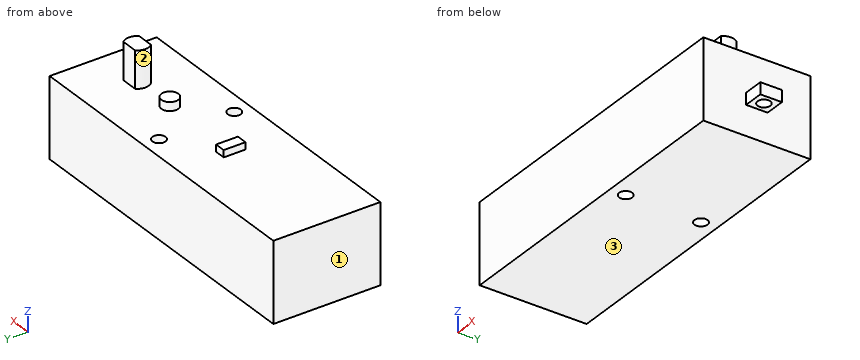
```python
from build123d import *

# Parameters (mm, degrees)
SKETCH1_W           = 75.1586
SKETCH1_H           = 25.1968
BOSS_EXTRUDE1_DEPTH = 18.7452
SKETCH2_W           = 4.8006
SKETCH2_H           = 5.08
BOSS_EXTRUDE2_DEPTH = 2.7432
SKETCH4_R           = 1.4986
CUT_EXTRUDE1_DEPTH  = 85.400741157
SKETCH3_R           = 1.9939
BOSS_EXTRUDE3_DEPTH = 2.032
SKETCH5_R           = 2.7051
BOSS_EXTRUDE4_DEPTH = 8.6614
CUT_EXTRUDE2_START  = -8.6614
CUT_EXTRUDE2_DEPTH  = 8.6614
SKETCH7_R           = 1.5367
CUT_EXTRUDE3_DEPTH  = 86.905383521
SKETCH8_W           = 2.54
SKETCH8_H           = 5.1308
BOSS_EXTRUDE5_DEPTH = 1.651


with BuildPart() as part:
    # Sketch1 → Boss-Extrude1 (new body)
    with BuildSketch(Plane.XY):
        with Locations((37.5793, 12.5984)):
            Rectangle(SKETCH1_W, SKETCH1_H)
    extrude(amount=BOSS_EXTRUDE1_DEPTH)

    # Sketch2 → Boss-Extrude2 (add)
    with BuildSketch(Plane.XY.offset(7.0104)):
        with Locations((77.5589, 12.5984)):
            Rectangle(SKETCH2_W, SKETCH2_H)
    extrude(amount=BOSS_EXTRUDE2_DEPTH)

    # Sketch4 → Cut-Extrude1 (cut, through all)
    with BuildSketch(Plane.XY.offset(9.7536)):
        with Locations((77.5589, 12.5984)):
            Circle(SKETCH4_R)
    extrude(amount=-CUT_EXTRUDE1_DEPTH, mode=Mode.SUBTRACT)

    # Sketch3 → Boss-Extrude3 (add)
    with BuildSketch(Plane.XY.offset(18.7452)):
        with Locations(Location((52.7431, 12.5984, 0), (0, 0, 180))):
            Circle(SKETCH3_R)
    extrude(amount=BOSS_EXTRUDE3_DEPTH)

    # Sketch5 → Boss-Extrude4 (add)
    with BuildSketch(Plane.XY.offset(18.7452)):
        with Locations(Location((63.7413, 12.5984, 0), (0, 0, 180))):
            Circle(SKETCH5_R)
    extrude(amount=BOSS_EXTRUDE4_DEPTH)

    # Sketch6 → Cut-Extrude2 (cut)
    with BuildSketch(Plane.XY.offset(27.4066).offset(CUT_EXTRUDE2_START)):
        with BuildLine():
            ThreePointArc((65.710946763, 14.4526), (63.7413, 15.3035), (61.771653237, 14.4526))
            Line((61.771653237, 14.4526), (65.710946763, 14.4526))
        make_face()
        with BuildLine():
            Line((65.710946763, 10.7442), (61.771653237, 10.7442))
            ThreePointArc((61.771653237, 10.7442), (63.7413, 9.8933), (65.710946763, 10.7442))
        make_face()
    extrude(amount=CUT_EXTRUDE2_DEPTH, mode=Mode.SUBTRACT)

    # Sketch7 → Cut-Extrude3 (cut, through all)
    with BuildSketch(Plane.XY.offset(18.7452)):
        with Locations((43.7515, 21.463)):
            Circle(SKETCH7_R)
        with Locations((43.7515, 3.7338)):
            Circle(SKETCH7_R)
    extrude(amount=-CUT_EXTRUDE3_DEPTH, mode=Mode.SUBTRACT)

    # Sketch8 → Boss-Extrude5 (add)
    with BuildSketch(Plane.XY.offset(18.7452)):
        with Locations((32.2707, 12.5984)):
            Rectangle(SKETCH8_W, SKETCH8_H)
    extrude(amount=BOSS_EXTRUDE5_DEPTH)


solid = part.part
```
Geometry check sheet. Reference: the model listing, model coordinates, mm. Face numbers are marked on the shaded views. Give positions to 0.01 mm unless a question says otherwise; leave off trailing zeros. Order: outer loops, then holes, each group sorted by start corner. A loop starts at its lowest first (then second) coordinate and runs counter-clockwise, first axis right, second up.
1. Section check B-B, the plane y = 20.75. Enter the section's corners in (x, z).
2. Release check for a two-part mould opening along X. For the marked faces 1, 2 and 3 record: pulls with the +X half, pulls with the -X half, needs draft (parallel to the pull), parting line crosses it, or undercut.
3. Section check A-A, the plane x = 65. Enter the section's corners in (y, z), and give its area (3 significant figures).
4. Section check D-D, the plane y = 16.5. Enter the section's corners in (x, z).
5. Gauge pin test, flat ends, axial feed: pin 1 Ø4 at (x, y) = (78, 13.5) entering from -Z; pin 2 Ø3 at (x, z) = (78.5, 9) entering from +Y; pin 3 Ø0.8 at (x, z) = (32, 20) entering from -Y; pin 4 Ø6 at (y, z) = (6.5, 10) entering from -X. Record the tip position at first contact, or that the pin passes through.
6. Thickness scan on L1, parallel to X at y = 7, z = 13; L2, parallel to Y at x = 62, z = 25.75; L3, parallel to Z at x = 28, y = 21. Record the ranges inside material, lowest first.
7. Section check C-C, the plane z = 10.5. Enter the section's corners in (x, y), and give its area (3 significant figures).
Values follow:
1. outline: (0, 0) - (42.39, 0) - (42.39, 18.75) - (0, 18.75) - close; (45.11, 0) - (75.16, 0) - (75.16, 18.75) - (45.11, 18.75) - close
2. face 1: pulls with the -X half
2. face 2: undercut
2. face 3: needs draft
3. outline: (0, 0) - (25.2, 0) - (25.2, 18.75) - (14.45, 18.75) - (14.45, 27.41) - (10.74, 27.41) - (10.74, 18.75) - (0, 18.75) - close
3. area: 504 mm2
4. outline: (0, 0) - (75.16, 0) - (75.16, 18.75) - (0, 18.75) - close
5. pin 1: stops at z = 7.01
5. pin 2: stops at y = 15.14
5. pin 3: stops at y = 10.03
5. pin 4: stops at x = 0
6. L1: x = 0 to 75.16
6. L2: y = 10.74 to 14.45
6. L3: z = 0 to 18.75
7. outline: (0, 0) - (75.16, 0) - (75.16, 25.2) - (0, 25.2) - close; hole circle Ø3.07 at (43.75, 3.73); hole circle Ø3.07 at (43.75, 21.46)
7. area: 1,880 mm2
